Geometry: final body of the model. Coordinates: model frame, mm. Round coordinates to 2 decimals unless told otherwise and drop trailing zeros. Loops run counter-clockwise (first coordinate to the right, second up) from the corner with the lowest first, then second, coordinate; pieces in that order, holes last. Notation, with made-up numbers: (-7, -23.75) - (52, -23.75) arc R22 cw to (52, -14.75) - close; hole circle Ø1 at (-2, -24). An arc over 180 degrees is marked (long way). Answer as a JSON object with one key per item and string values. Group by question number.
Item 1: Section A-A (x = 90.17). Return the cut outline in (y, z), plus the area to 3 significant figures.
Item 2: First-contact query: pin 1 (0.8 mm diameter, centred on y = 44.5, z = 0.5, fed in from +X). Flat tip, straight axial feed; report the tip coordinate or a pass-through.
Item 3: Section C-C (x = 66.04). Return the cut outline in (y, z).
Item 4: Draft query along X for faces 1 (the face through (50, 27, 1.588)), 2 (the face through (97.61, 52.11, 0.78)), 3 (the face through (67.506, 34.952, 0.783)). Return one class per face: released by +X, released by -X, zero draft, split by the parting line, or undercut.
Item 5: Line query: line 1 (Y direction, x = 90.17, z = 0.4); line 2 (Y direction, x = 13.97, z = 0.8); line 3 (Y direction, x = 65, z = 1.1). Output: solid intervals per line, ascending.
Item 6: Section B-B (y = 35.56). Return the cut outline in (x, z), plus the area to 3 significant figures.
Item 7: Section D-D (y = 43.5). Return the cut outline in (x, z), plus the area to 3 significant figures.
```python
from build123d import *

# Parameters (mm, degrees)
SKETCH1_R           = 1.5875
BOSS_EXTRUDE1_DEPTH = 1.5875


with BuildPart() as part:
    # Sketch1 → Boss-Extrude1 (new body)
    with BuildSketch(Plane.XY):
        Polygon((0, 53.34), (0, 0), (98.806, 0), (98.806, 1.27), (101.6, 4.064), (101.6, 38.354), (98.806, 41.148), (98.806, 50.915330847), (96.381330847, 53.34), align=None)
        with Locations((13.97, 2.54)):
            Circle(SKETCH1_R, mode=Mode.SUBTRACT)
        with Locations((66.04, 7.62)):
            Circle(SKETCH1_R, mode=Mode.SUBTRACT)
        with Locations((96.266, 2.54)):
            Circle(SKETCH1_R, mode=Mode.SUBTRACT)
        with Locations((15.24, 50.8)):
            Circle(SKETCH1_R, mode=Mode.SUBTRACT)
        with Locations((66.04, 35.56)):
            Circle(SKETCH1_R, mode=Mode.SUBTRACT)
        with Locations((90.17, 50.8)):
            Circle(SKETCH1_R, mode=Mode.SUBTRACT)
    extrude(amount=BOSS_EXTRUDE1_DEPTH)


solid = part.part
```
Values:
{
 "1": {"outline": "(0, 0) - (49.21, 0) - (49.21, 1.59) - (0, 1.59) - close; (52.39, 0) - (53.34, 0) - (53.34, 1.59) - (52.39, 1.59) - close", "area": "79.6 mm^2"},
 "2": {"pin 1": "stops at x = 98.81"},
 "3": {"outline": "(0, 0) - (6.03, 0) - (6.03, 1.59) - (0, 1.59) - close; (9.21, 0) - (33.97, 0) - (33.97, 1.59) - (9.21, 1.59) - close; (37.15, 0) - (53.34, 0) - (53.34, 1.59) - (37.15, 1.59) - close"},
 "4": {"face 1": "zero draft", "face 2": "released by +X", "face 3": "undercut"},
 "5": {"line 1": "y = 0 to 49.21, 52.39 to 53.34", "line 2": "y = 0 to 0.95, 4.13 to 49.85, 51.75 to 53.34", "line 3": "y = 0 to 6.42, 8.82 to 34.36, 36.76 to 53.34"},
 "6": {"outline": "(0, 0) - (64.45, 0) - (64.45, 1.59) - (0, 1.59) - close; (67.63, 0) - (101.6, 0) - (101.6, 1.59) - (67.63, 1.59) - close", "area": "156 mm^2"},
 "7": {"outline": "(0, 0) - (98.81, 0) - (98.81, 1.59) - (0, 1.59) - close", "area": "157 mm^2"}
}
